Model file for the job. Use its own axes, mm. A direction names the side the tool comes from. Give positions to 0.01 mm unless a question says otherwise; leave off trailing zeros. Write each loop counter-clockwise with the first axis right and the second up, starting at its lowest first coordinate (ties: lowest second). Pieces come first, ordered by that corner, then holes. Notation, with made-up numbers: M 4,40 L 36,40 A23 ccw 36,63 Z; hole C 36.25,77 d10. An arc over 180 degrees is marked long. Answer as a JSON object with one key per item and string values. Group by question number.
```python
from build123d import *
from build123d.topology import SkipClean

# Parameters (mm, degrees)
SKETCH1_W           = 18
SKETCH1_H           = 22
BOSS_EXTRUDE1_DEPTH = 36.5
FILLET1_R           = 4
BOSS_EXTRUDE2_DEPTH = 11.5
BOSS_EXTRUDE3_DEPTH = 2
SKETCH4_W           = 6
SKETCH4_H           = 1.5
CUT_EXTRUDE1_DEPTH  = 4
FILLET2_R           = 0.4
FILLET3_R           = 0.4
FILLET4_R           = 0.4
SKETCH5_R           = 1.5
CUT_EXTRUDE2_DEPTH  = 54.150729064
SKETCH5_3_R         = 1.5
SKETCH5_3_R_2       = 2.45
SKETCH5_3_R_3       = 2
CUT_EXTRUDE3_DEPTH  = 1
SKETCH6_R           = 0.75
CUT_EXTRUDE4_DEPTH  = 9
SKETCH7_R           = 0.75
CUT_EXTRUDE5_DEPTH  = 8
SKETCH8_R           = 2.5
CUT_EXTRUDE6_DEPTH  = 54.150729064
BOSS_EXTRUDE4_START = 0.125
SKETCH8_3_R         = 3
SKETCH8_3_R_2       = 2.5
BOSS_EXTRUDE4_DEPTH = 0.125
SKETCH11_R          = 1.5
BOSS_EXTRUDE5_DEPTH = 1.25


with BuildPart() as part:
    # Sketch1 → Boss-Extrude1 (new body)
    with BuildSketch(Plane(origin=(0, 0, 0), x_dir=(1, 0, 0), z_dir=(0, 1, 0))):
        Rectangle(SKETCH1_W, SKETCH1_H)
    extrude(amount=BOSS_EXTRUDE1_DEPTH)

    # Fillet1
    fillet1_edges = [part.edges().sort_by_distance(p)[0] for p in [
        (0, 0, 11),
        (0, 0, -11),
    ]]
    fillet(fillet1_edges, radius=FILLET1_R)

    # Sketch2 → Boss-Extrude2 (add)
    with BuildSketch(Plane(origin=(0, 36.5, 0), x_dir=(1, 0, 0), z_dir=(0, 1, 0))):
        with BuildLine():
            Line((-9, 6.32455532), (-9, -6.32455532))
            ThreePointArc((-9, -6.32455532), (0, -11), (9, -6.32455532))
            Line((9, -6.32455532), (9, 6.32455532))
            ThreePointArc((9, 6.32455532), (0, 11), (-9, 6.32455532))
        make_face()
        with BuildLine():
            Line((-8, 6), (-8, -6))
            ThreePointArc((-8, -6), (0, -10), (8, -6))
            Line((8, -6), (8, 6))
            ThreePointArc((8, 6), (0, 10), (-8, 6))
        make_face(mode=Mode.SUBTRACT)
    extrude(amount=BOSS_EXTRUDE2_DEPTH)

    # Sketch3 → Boss-Extrude3 (add, symmetric)
    with BuildSketch(Plane.XY):
        Polygon((-9, 45), (-10.5, 45), (-10.5, 43.5), (-11, 43.5), (-11, 45.5), (-9, 45.5), align=None)
    boss_extrude3 = extrude(amount=BOSS_EXTRUDE3_DEPTH, both=True)

    # Sketch4 → Cut-Extrude1 (cut)
    with BuildSketch(Plane.ZY.offset(9)):
        with Locations((0, 44.25)):
            Rectangle(SKETCH4_W, SKETCH4_H)
    cut_extrude1 = extrude(amount=-CUT_EXTRUDE1_DEPTH, mode=Mode.SUBTRACT)

    # Fillet2
    fillet2_edges = [part.edges().sort_by_distance(p)[0] for p in [
        (-9, 45.25, -2),
        (-9, 45.5, 0),
        (-9, 45.25, 2),
    ]]
    fillet(fillet2_edges, radius=FILLET2_R)

    # Fillet3
    fillet3_edges = [part.edges().sort_by_distance(p)[0] for p in [
        (-11, 45.5, 0),
    ]]
    fillet(fillet3_edges, radius=FILLET3_R)

    # Mirror1: Boss-Extrude3, Cut-Extrude1 across plane
    add(boss_extrude3.mirror(Plane(origin=(0, 0, 0), x_dir=(0, 0, 1), z_dir=(1, 0, 0))))
    add(cut_extrude1.mirror(Plane(origin=(0, 0, 0), x_dir=(0, 0, 1), z_dir=(1, 0, 0))), mode=Mode.SUBTRACT)

    # Fillet4
    fillet4_edges = [part.edges().sort_by_distance(p)[0] for p in [
        (9, 45.25, 2),
        (9, 45.5, 0),
        (11, 45.5, 0),
        (9, 45.25, -2),
    ]]
    fillet(fillet4_edges, radius=FILLET4_R)

    # Sketch5 → Cut-Extrude2 (cut, through all)
    with BuildSketch(Plane.ZY.offset(9)):
        with Locations((9, 31.5)):
            Circle(SKETCH5_R)
    cut_extrude2 = extrude(amount=-CUT_EXTRUDE2_DEPTH, mode=Mode.SUBTRACT)

    # Sketch5<3> → Cut-Extrude3 (cut)
    # profile 1 of 5: a face of its own
    with BuildSketch(Plane.ZY.offset(9)):
        with Locations((9, 31.5)):
            Circle(SKETCH5_3_R)
    # profile 2 of 5: a face of its own
    with BuildSketch(Plane.ZY.offset(9)):
        with Locations((6, 34)):
            Circle(SKETCH5_3_R_2)
        with Locations((6, 34)):
            Circle(SKETCH5_3_R_3, mode=Mode.SUBTRACT)
    # profile 3 of 5: a face of its own
    with BuildSketch(Plane.ZY.offset(9)):
        with Locations((6, 34)):
            Circle(SKETCH5_3_R_3)
    # profile 4 of 5: a face of its own
    with BuildSketch(Plane.ZY.offset(9)):
        with Locations((9, 31.5)):
            Circle(SKETCH5_3_R)
    # profile 5 of 5: a face of its own
    with BuildSketch(Plane.ZY.offset(9)):
        with Locations((6, 34)):
            Circle(SKETCH5_3_R_2)
    cut_extrude3 = extrude(amount=-CUT_EXTRUDE3_DEPTH, mode=Mode.SUBTRACT)

    # Sketch6 → Cut-Extrude4 (cut)
    with BuildSketch(Plane.ZY.offset(8)):
        with Locations((6, 34)):
            Circle(SKETCH6_R)
    cut_extrude4 = extrude(amount=-CUT_EXTRUDE4_DEPTH, mode=Mode.SUBTRACT)

    # Mirror4: Cut-Extrude2, Cut-Extrude3, Cut-Extrude4 across plane
    add(cut_extrude2.mirror(Plane.XY), mode=Mode.SUBTRACT)
    add(cut_extrude3.mirror(Plane.XY), mode=Mode.SUBTRACT)
    add(cut_extrude4.mirror(Plane.XY), mode=Mode.SUBTRACT)

    # Sketch7 → Cut-Extrude5 (cut)
    with BuildSketch(Plane(origin=(9, 0, 0), x_dir=(0, 0, -1), z_dir=(1, 0, 0))):
        with Locations((-9.75, 35.25)):
            Circle(SKETCH7_R)
    cut_extrude5 = extrude(amount=-CUT_EXTRUDE5_DEPTH, mode=Mode.SUBTRACT)

    # Mirror5: Cut-Extrude5 across plane
    add(cut_extrude5.mirror(Plane.XY), mode=Mode.SUBTRACT)

    # Sketch8 → Cut-Extrude6 (cut, through all)
    with BuildSketch(Plane.ZY.offset(9)):
        with Locations((0, 11)):
            Circle(SKETCH8_R)
    extrude(amount=-CUT_EXTRUDE6_DEPTH, mode=Mode.SUBTRACT)

    # Sketch8<3> → Boss-Extrude4 (add)
    with BuildSketch(Plane.ZY.offset(9).offset(BOSS_EXTRUDE4_START)):
        with Locations(Location((0, 11, 0), (0, 0, 180))):
            Circle(SKETCH8_3_R)
        with Locations((0, 11)):
            Circle(SKETCH8_3_R_2, mode=Mode.SUBTRACT)
    boss_extrude4 = extrude(amount=-BOSS_EXTRUDE4_DEPTH)

    # Sketch9 → Revolve1 (revolve)
    with SkipClean():  # the faces are left unmerged after this step: merging them gives an invalid solid
        with BuildSketch(Plane(origin=(0, 22, 0), x_dir=(-1, 0, 0), z_dir=(0, -1, 0))):
            with BuildLine():
                Line((9, 1.5), (9, -1.5))
                ThreePointArc((9, -1.5), (10.5, 0), (9, 1.5))
            make_face()
        revolve(axis=Axis((-9, 22, -1.5), (0, 0, 1)))

    # Mirror6: Boss-Extrude4 across plane
    with SkipClean():  # the faces are left unmerged after this step: merging them gives an invalid solid
        add(boss_extrude4.mirror(Plane(origin=(0, 0, 0), x_dir=(0, 0, 1), z_dir=(1, 0, 0))))

    # Sketch11 → Boss-Extrude5 (add, symmetric)
    with SkipClean():  # the faces are left unmerged after this step: merging them gives an invalid solid
        with BuildSketch(Plane(origin=(0, 0, 0), x_dir=(0, 0, -1), z_dir=(1, 0, 0))):
            Polygon((-2.5, -2.810816006), (-2.5, 0), (2.5, 0), (2.5, -2.810816006), (2.5, -5), (-2.5, -5), align=None)
            with Locations((0, -2.5)):
                Circle(SKETCH11_R, mode=Mode.SUBTRACT)
        extrude(amount=BOSS_EXTRUDE5_DEPTH, both=True)


solid = part.part
```
Q1. 3-axis set-ups, long thin cutter, end or side, ignore diameter. For faces 1 (the flat face through (-7, 36.5, -10)), 2 (the flat face through (-7, 36.5, 10)), 3 (the flat face through (-8.5, 43.5, 0)), 4 (the flat face through (-10, 45.5, 0)), 5 (the cylindrical face through (0, 42, -11)): which of +Z, -Z, +X, -X, +Y, -Y reach the whole face in a straight line?
Q2. Slice it at C-C, the plane x = 0.5. Count the separate pieces of the cut face and the enclosed holes in it, then the cut area to 3 significant figures.
Q3. Slice it at B-B, the plane y = -2.5. Write the cut outline in (x, z), then the cut area to 3 significant figures.
Q4. Slice it at A-A, the plane y = 40. Write the cut outline in (x, z), then the cut area to 3 significant figures.
Q5. Two-plate mould, pull along X, no slides. Class faces 6 (the cylindrical face through (-8.51, 35.65, -4.19)), 7 (the flat face through (-1.25, -1, 1)), 8 (the flat face through (-8, 42, 0)): +X half, -X half, draft (parallel to the pull), parting line (faces both ways), or undercut.
Q6. Slice it at D-D, the plane x = 7.5. Write the cut outline in (y, z).
Q7. Wall check: L1, parallel to Z at x = -4.5, y = 34; L2, parallel to Z at x = 3, y = 35.25; L3, parallel to Y at x = 0.7, z = 0. Give the ranges that are in metal, low to high.
Q8. Drop flat-ended pins along their axis: P1, Ø1.1, axis at x = -8.5, y = 44.5, coming from the +Z side; P2, Ø1, axis at x = -8.5, z = -8.5, coming from the -Y side; P3, Ø0.6, axis at x = 10, z = -1, coming from the +Y side; P4, Ø8, axis at x = 7, y = 40, coming from the -Z side. Give the stop position or say it passes through.
Solved:
{
 "1": {"face 1": "-Z, -X, +Y", "face 2": "+Z, -X, +Y", "face 3": "none", "face 4": "+Z, -Z, -X, +Y", "face 5": "-Z, +Y"},
 "2": {"separate pieces": "1", "enclosed holes": "6", "area": "800 mm²"},
 "3": {"outline": "M -1.25,-2.5 L 1.25,-2.5 L 1.25,-1.5 L -1.25,-1.5 Z; M -1.25,1.5 L 1.25,1.5 L 1.25,2.5 L -1.25,2.5 Z", "area": "5.00 mm²"},
 "4": {"outline": "M -9,-6.32 A11 ccw 9,-6.32 L 9,6.32 A11 ccw -9,6.32 Z; hole M -8,-6 A10 ccw 8,-6 L 8,6 A10 ccw -8,6 Z", "area": "64.3 mm²"},
 "5": {"face 6": "draft", "face 7": "-X half", "face 8": "undercut"},
 "6": {"outline": "M 0,-7 A4 ccw 4,-11 L 36.5,-11 L 36.5,-8.05 L 48,-8.05 L 48,-6.61 L 36.5,-6.61 L 36.5,6.61 L 48,6.61 L 48,8.05 L 36.5,8.05 L 36.5,11 L 4,11 A4 ccw 0,7 Z; hole C 11,0 d5; hole C 31.5,-9 d3; hole C 31.5,9 d3; hole C 35.25,-9.75 d1.5; hole C 35.25,9.75 d1.5"},
 "7": {"L1": "z = -11 to -6.75, -5.25 to 5.25, 6.75 to 11", "L2": "z = -11 to -10.5, -9 to 9, 10.5 to 11", "L3": "y = -5 to -4, -1 to 8.5, 13.5 to 36.5"},
 "8": {"P1": "stops at z = 7.6", "P2": "stops at y = 0.13", "P3": "stops at y = 45.5", "P4": "stops at z = -11"}
}
